Here's how the part is built. I have some questions about the finished solid (model axes, mm). Face numbers are marked on the shaded views. A direction names the side the tool comes from. Give positions to 0.01 mm unless a question says otherwise; leave off trailing zeros. Loops run counter-clockwise (first coordinate to the right, second up) from the corner with the lowest first, then second, coordinate; pieces in that order, holes last. Notation, with made-up numbers: (10.5, -6.5) - (67.5, -6.5) arc R24 cw to (67.5, 7.5) - close; hole circle Ø4 at (21, 50.5). An arc over 180 degrees is marked (long way). Put each result on its own line as item: value. Start each with the question number.
from build123d import *

# Parameters (mm, degrees)
PAD_DEPTH       = 8
SKETCH003_W     = 23.2
SKETCH003_H     = 17.2
POCKET_DEPTH    = 6
SKETCH005_W     = 2.2
SKETCH005_H     = 8.4
POCKET001_DEPTH = 7
SKETCH006_W     = 4.2
SKETCH006_H     = 4.2
POCKET002_DEPTH = 5
SKETCH007_W     = 4
SKETCH007_H     = 4
PAD001_DEPTH    = 6
SKETCH008_W     = 4
SKETCH008_H     = 4
PAD002_DEPTH    = 6


with BuildPart() as part:
    # Sketch → Pad (new body)
    with BuildSketch(Plane.XY):
        Polygon((-4, 14.6), (-4, 10.6), (0, 10.6), (0, 0), (31.8, 0), (31.8, 10.6), (35.8, 10.6), (35.8, 14.6), (31.8, 14.6), (31.8, 25.2), (0, 25.2), (0, 14.6), align=None)
    extrude(amount=PAD_DEPTH)

    # Sketch003 (on DatumPlane) → Pocket (cut)
    with BuildSketch(Plane.XY.offset(8)):
        with Locations((18.2, 12.6)):
            Rectangle(SKETCH003_W, SKETCH003_H)
    extrude(amount=-POCKET_DEPTH, mode=Mode.SUBTRACT)

    # Sketch005 (on DatumPlane) → Pocket001 (cut)
    with BuildSketch(Plane.XY.offset(2)):
        with Locations((9.7, 12.6)):
            Rectangle(SKETCH005_W, SKETCH005_H)
    extrude(amount=-POCKET001_DEPTH, mode=Mode.SUBTRACT)

    # Sketch006 (on DatumPlane) → Pocket002 (cut)
    with BuildSketch(Plane.XY.offset(2)):
        with Locations((21.2, 12.6)):
            Rectangle(SKETCH006_W, SKETCH006_H)
    extrude(amount=-POCKET002_DEPTH, mode=Mode.SUBTRACT)

    # Sketch007 (on DatumPlane) → Pad001 (join)
    with BuildSketch(Plane.XY.offset(8)):
        with Locations((-2, 12.6)):
            Rectangle(SKETCH007_W, SKETCH007_H)
    extrude(amount=PAD001_DEPTH)

    # Sketch008 (on DatumPlane) → Pad002 (join)
    with BuildSketch(Plane.XY.offset(8)):
        with Locations((33.8, 12.6)):
            Rectangle(SKETCH008_W, SKETCH008_H)
    extrude(amount=PAD002_DEPTH)


solid = part.part
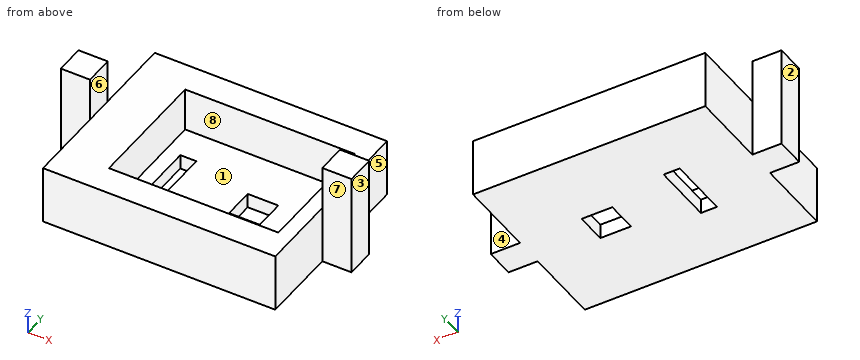
1) I'm going to push flat-ended pins straight in: P1, Ø1.5, axis at x = 28, y = 14, coming from the +Z side; P2, Ø1.2, axis at x = -1.5, z = 10.5, coming from the +Y side; P3, Ø6.5, axis at y = 15, z = 6, coming from the +X side; P4, Ø6.5, axis at y = 20.5, z = 2, coming from the -X side. Where does each tip first touch, or does it pass through?
2) Thinking about a two-plate mould opening in X: for the marked faces 1, 2, 3 and 4, which applies, pulls with the +X half, pulls with the -X half, needs draft (parallel to the pull), parting line crosses it, or undercut?
3) Which directions (+Z, -Z, +X, -X, +Y, -Y) give clear straight access to the entire face, cutting with the end or side of a thin tool? Please do the marked faces 5, 6, 7 and 8.
4) I need wall thicknesses on line 1 (Y direction, x = 12, z = 4); line 2 (X direction, y = 8.75, z = 6); line 3 (X direction, y = 11.5, z = 10). Which ranges of each line are inside material? Lowest first, please.
5) Suppose I cut it at C-C on x = 24. Please give me the cut outline in (y, z), plus the area to 3 significant figures.
6) Suppose I cut it at A-A on z = 2.75. Please give me the cut outline in (x, y), plus the area to 3 significant figures.
7) Suppose I cut it at D-D on y = 7. Please give me the cut outline in (x, z), plus the area to 3 significant figures.
8) Suppose I cut it at B-B on z = 8.5. Please give me the cut outline in (x, y), plus the area to 3 significant figures.
Ans:
1. P1: stops at z = 2
1. P2: stops at y = 14.6
1. P3: stops at x = 35.8
1. P4: stops at x = 0
2. face 1: undercut
2. face 2: pulls with the -X half
2. face 3: pulls with the +X half
2. face 4: needs draft
3. face 5: +Z, -Z, +X, +Y
3. face 6: +Z, +Y, -Y
3. face 7: +Z, -Z, +X, -Y
3. face 8: +Z
4. line 1: y = 0 to 4, 21.2 to 25.2
4. line 2: x = 0 to 6.6, 29.8 to 31.8
4. line 3: x = -4 to 0, 31.8 to 35.8
5. outline: (0, 0) - (25.2, 0) - (25.2, 8) - (21.2, 8) - (21.2, 2) - (4, 2) - (4, 8) - (0, 8) - close
5. area: 98.4 mm²
6. outline: (-4, 10.6) - (0, 10.6) - (0, 0) - (31.8, 0) - (31.8, 10.6) - (35.8, 10.6) - (35.8, 14.6) - (31.8, 14.6) - (31.8, 25.2) - (0, 25.2) - (0, 14.6) - (-4, 14.6) - close; hole (6.6, 4) - (29.8, 4) - (29.8, 21.2) - (6.6, 21.2) - close
6. area: 434 mm²
7. outline: (0, 0) - (31.8, 0) - (31.8, 8) - (29.8, 8) - (29.8, 2) - (6.6, 2) - (6.6, 8) - (0, 8) - close
7. area: 115 mm²
8. outline: (-4, 10.6) - (0, 10.6) - (0, 14.6) - (-4, 14.6) - close; (31.8, 10.6) - (35.8, 10.6) - (35.8, 14.6) - (31.8, 14.6) - close
8. area: 32.0 mm²
